Geometry: final body of the model. Coordinates: model frame, mm. A direction names the side the tool comes from. Give positions to 0.01 mm unless a question says otherwise; leave off trailing zeros. Loops run counter-clockwise (first coordinate to the right, second up) from the corner with the lowest first, then second, coordinate; pieces in that order, holes last.
from build123d import *

# Parameters (mm, degrees)
F1_DEPTH = 12.7
F2_DEPTH = 12.7
F4_DEPTH = 25.4


with BuildPart() as f1:
    # F0 (on Front) → F1 (new body)
    with BuildSketch(Plane.XZ):
        with BuildLine():
            ThreePointArc((-62.636777, 25.519665), (-75.336777, 38.219665), (-88.036777, 25.519665))
            Line((-88.036777, 25.519665), (-81.686777, 25.519665))
            ThreePointArc((-81.686777, 25.519665), (-75.336777, 31.869665), (-68.986777, 25.519665))
            Line((-68.986777, 25.519665), (-62.636777, 25.519665))
        make_face()
        with BuildLine():
            Line((-81.686777, 25.519665), (-88.036777, 25.519665))
            Line((-88.036777, 25.519665), (-88.036777, -6.230335))
            Line((-88.036777, -6.230335), (-62.636777, -6.230335))
            Line((-62.636777, -6.230335), (-62.636777, 0.119665))
            Line((-62.636777, 0.119665), (-62.636777, 12.819665))
            Line((-62.636777, 12.819665), (-62.636777, 25.519665))
            Line((-62.636777, 25.519665), (-68.986777, 25.519665))
            ThreePointArc((-68.986777, 25.519665), (-75.336777, 19.169665), (-81.686777, 25.519665))
        make_face()
    extrude(amount=F1_DEPTH)

    # F0 (on Front) → F2 (join)
    with BuildSketch(Plane.XZ):
        with BuildLine():
            Line((-81.686777, 25.519665), (-88.036777, 25.519665))
            Line((-88.036777, 25.519665), (-88.036777, -6.230335))
            Line((-88.036777, -6.230335), (-62.636777, -6.230335))
            Line((-62.636777, -6.230335), (-62.636777, 0.119665))
            Line((-62.636777, 0.119665), (-62.636777, 12.819665))
            Line((-62.636777, 12.819665), (-62.636777, 25.519665))
            Line((-62.636777, 25.519665), (-68.986777, 25.519665))
            ThreePointArc((-68.986777, 25.519665), (-75.336777, 19.169665), (-81.686777, 25.519665))
        make_face()
        with BuildLine():
            ThreePointArc((-62.636777, 25.519665), (-75.336777, 38.219665), (-88.036777, 25.519665))
            Line((-88.036777, 25.519665), (-81.686777, 25.519665))
            ThreePointArc((-81.686777, 25.519665), (-75.336777, 31.869665), (-68.986777, 25.519665))
            Line((-68.986777, 25.519665), (-62.636777, 25.519665))
        make_face()
        Polygon((-62.636777, 0.119665), (-62.636777, -6.230335), (-24.536777, -6.230335), (-24.536777, 0.119665), (-49.936777, 0.119665), align=None)
        with BuildLine():
            ThreePointArc((-49.936777, 0.119665), (-57.818406, 4.938036), (-62.636777, 12.819665))
            Line((-62.636777, 12.819665), (-62.636777, 0.119665))
            Line((-62.636777, 0.119665), (-49.936777, 0.119665))
        make_face()
    extrude(amount=F2_DEPTH)

    # F3 (on face) → F4 (join)
    with BuildSketch(Plane.XZ.offset(12.7)):
        Polygon((-24.536777, -6.230335), (-24.536777, 0.119665), (-49.936777, 0.119665), (-88.036777, 0.119665), (-88.036777, -6.230335), align=None)
    extrude(amount=F4_DEPTH)


solid = f1.part
Item 1: Set-up query: faces 1 (the face through (-56, -23, 0.12)), 2 (the face through (-71, 0, 11)), 3 (the face through (-62.637, -6, 19)). Return all of +Z, -Z, +X, -X, +Y, -Y with unobstructed straight access to the full face (end or side cutting, diameter ignored); none if empty.
Values follow:
face 1: +Z, +X, -Y
face 2: +Z, -Z, +X, -X, +Y
face 3: +Z, +X, +Y, -Y
Item 2: Pin query (flat end, axial travel): pin 1 (14.5 mm diameter, centred on x = -75.34, z = 25.52, fed in from -Y); pin 2 (8 mm diameter, centred on x = -80, y = -32.5, fed in from +Z); pin 3 (4 mm diameter, centred on y = -5, z = 22, fed in from +X). Return the tip coordinate at first contact, or that it passes through.
Values follow:
pin 1: stops at y = -12.7
pin 2: stops at z = 0.12
pin 3: stops at x = -62.64
Item 3: Draft query along X for faces 4 (the face through (-73, -12.7, 15)), 5 (the face through (-24.537, -19, -3)), 6 (the face through (-71.923, -6.261, 20.165)). Return one class per face: +X half, -X half, draft (parallel to the pull), parting line (faces both ways), or undercut.
Values follow:
face 4: draft
face 5: +X half
face 6: undercut
Item 4: Section query B-B on x = -70. Return loops of the section in (y, z), plus the area to 3 significant figures.
Values follow:
outline: (-38.1, -6.23) - (0, -6.23) - (0, 22.08) - (-12.7, 22.08) - (-12.7, 0.12) - (-38.1, 0.12) - close; (-12.7, 28.96) - (0, 28.96) - (0, 37.04) - (-12.7, 37.04) - close
area: 623 mm2
Item 5: Section query D-D on x = -48.5. Return loops of the section in (y, z), plus the area to 3 significant figures.
Values follow:
outline: (-38.1, -6.23) - (0, -6.23) - (0, 0.12) - (-38.1, 0.12) - close
area: 242 mm2
Item 6: Section query C-C on z = 22.5. Return loops of the section in (x, y), plus the area to 3 significant figures.
Values follow:
outline: (-88.04, -12.7) - (-80.92, -12.7) - (-80.92, 0) - (-88.04, 0) - close; (-69.75, -12.7) - (-62.64, -12.7) - (-62.64, 0) - (-69.75, 0) - close
area: 181 mm2
Item 7: Section query A-A on y = -12. Return loops of the section in (x, z).
Values follow:
outline: (-88.04, -6.23) - (-24.54, -6.23) - (-24.54, 0.12) - (-49.94, 0.12) arc R19.7 cw to (-62.64, 12.82) - (-62.64, 25.52) arc R12.7 ccw to (-88.04, 25.52) - close; hole circle Ø12.7 at (-75.34, 25.52)
Item 8: Ray query, probe 1 along Y at (x, z) = (-68.5, 4); probe 2 along X at (y, z) = (-4, 15); probe 3 along Z at (x, y) = (-34, -7). Return the intervals inside material, ascending.
Values follow:
probe 1: y = -12.7 to 0
probe 2: x = -88.04 to -62.64
probe 3: z = -6.23 to 0.12
